Read the model definition and answer for the solid it produces. Units are mm, in the model's axes. Face numbers are marked on the shaded views. A direction names the side the tool comes from. Coordinates: 2 decimals unless noted, no trailing zeros. Loops run counter-clockwise (first coordinate to the right, second up) from the corner with the lowest first, then second, coordinate; pieces in that order, holes last.
Q1. Flat-ended cylindrical pins translate along their axes: P1, Ø1, axis at x = -11, y = -6, coming from the +Z side; P2, Ø5, axis at x = 12.5, y = -3, coming from the -Z side; P3, Ø0.9, axis at x = -21, y = 6.5, coming from the +Z side. Find the tip coordinate at first contact, or state that the pin passes through.
Q2. Section A-A (y = 0) is taken. Give the vertices of the cut face in (x, z) (3 decimals).
Q3. The mould has two halves that part along X. Classify the marked faces 1, 2 and 3: pulls with the +X half, pulls with the -X half, needs draft (parallel to the pull), parting line crosses it, or undercut.
Q4. Which of the six approach directions +Z, -Z, +X, -X, +Y, -Y give full straight-line access (tool end or side, diameter ignored) to the marked faces 4 and 5?
Q5. Section B-B (z = 0) is taken. Give the vertices of the cut face in (x, y) (3 decimals), then the cut area to 3 significant figures.
Q6. Section C-C (x = 24) is taken. Give the vertices of the cut face in (y, z).
Q7. Straight lines are drawn through the part: line 1 (X direction, y = 3.5, z = -4.25); line 2 (Z direction, x = 9, y = 0); line 3 (Z direction, x = 15.5, y = 0). For each, find the intervals that lie inside material, in ascending order.
Q8. Section D-D (z = 6) is taken. Give the vertices of the cut face in (x, y).
from build123d import *

# Parameters (mm, degrees)
F0_R      = 9
F1_DEPTH  = 14
F2_R      = 7.5
F3_DEPTH  = 15
F4_R      = 5
F5_DEPTH  = 10
F6_R      = 7.5
F7_DEPTH  = 11.5
F8_R      = 7.425
F9_DEPTH  = 1.5
F10_R     = 8
F11_DEPTH = 2
F13_DEPTH = 13.5


with BuildPart() as f1:
    # F0 (on Right) → F1 (new body, symmetric)
    with BuildSketch(Plane.YZ):
        Circle(F0_R)
    extrude(amount=F1_DEPTH, both=True)

    # F2 (on face) → F3 (join)
    with BuildSketch(Plane.YZ.offset(14)):
        Circle(F2_R)
    extrude(amount=F3_DEPTH)

    # F4 (on face) → F5 (join)
    with BuildSketch(Plane.YZ.offset(29)):
        Circle(F4_R)
    extrude(amount=F5_DEPTH)

    # F6 (on face) → F7 (join)
    with BuildSketch(Plane(origin=(-14, 0, 0), x_dir=(0, -1, 0), z_dir=(-1, 0, 0))):
        Circle(F6_R)
    extrude(amount=F7_DEPTH)

    # F8 (on face) → F9 (join)
    with BuildSketch(Plane(origin=(-25.5, 0, 0), x_dir=(0, -1, 0), z_dir=(-1, 0, 0))):
        Circle(F8_R)
    extrude(amount=F9_DEPTH)

    # F10 (on face) → F11 (join)
    with BuildSketch(Plane(origin=(-27, 0, 0), x_dir=(0, -1, 0), z_dir=(-1, 0, 0))):
        Circle(F10_R)
    extrude(amount=F11_DEPTH)

    # F12 (on face) → F13 (cut)
    with BuildSketch(Plane(origin=(-29, 0, 0), x_dir=(0, -1, 0), z_dir=(-1, 0, 0))):
        with BuildLine():
            Line((-7.8581168228, -1.5), (-4.8581168228, -1.5))
            Line((-4.8581168228, -1.5), (-4.8581168228, 1.5))
            Line((-4.8581168228, 1.5), (-7.8581168228, 1.5))
            add(Edge.make_bspline(
                [(-7.8581168228, 1.5), (-8.0546390686, 1), (-8.4476835604, 0), (-8.0546390686, -1), (-7.8581168228, -1.5)],
                knots=[0, 0, 0, 0, 0.5, 1, 1, 1, 1], degree=3))
        make_face()
    extrude(amount=-F13_DEPTH, mode=Mode.SUBTRACT)


solid = f1.part
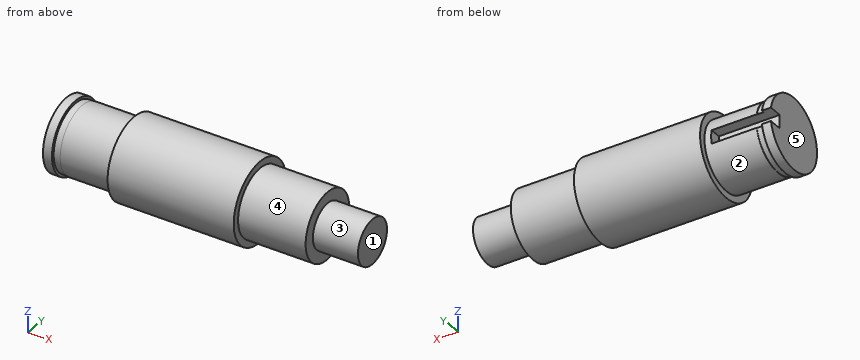
Numbers:
1. P1: stops at z = 7.12
1. P2: stops at z = -8.99
1. P3: stops at z = 4.43
2. outline: (-29, -8) - (-27, -8) - (-27, -7.425) - (-25.5, -7.425) - (-25.5, -7.5) - (-14, -7.5) - (-14, -9) - (14, -9) - (14, -7.5) - (29, -7.5) - (29, -5) - (39, -5) - (39, 5) - (29, 5) - (29, 7.5) - (14, 7.5) - (14, 9) - (-14, 9) - (-14, 7.5) - (-25.5, 7.5) - (-25.5, 7.425) - (-27, 7.425) - (-27, 8) - (-29, 8) - close
3. face 1: pulls with the +X half
3. face 2: undercut
3. face 3: needs draft
4. face 4: +X
4. face 5: +Z, -Z, -X, +Y, -Y
5. outline: (-29, -8) - (-27, -8) - (-27, -7.425) - (-25.5, -7.425) - (-25.5, -7.5) - (-14, -7.5) - (-14, -9) - (14, -9) - (14, -7.5) - (29, -7.5) - (29, -5) - (39, -5) - (39, 5) - (29, 5) - (29, 7.5) - (14, 7.5) - (14, 9) - (-14, 9) - (-14, 7.5) - (-15.5, 7.5) - (-15.5, 4.858) - (-29, 4.858) - close
5. area: 1,020 mm2
6. outline: circle Ø15 at (0, 0)
7. line 1: x = -29 to 29
7. line 2: z = -9 to 9
7. line 3: z = -7.5 to 7.5
8. outline: (-29, -5.29) - (-27, -5.29) - (-27, -4.37) - (-25.5, -4.37) - (-25.5, -4.5) - (-14, -4.5) - (-14, -6.71) - (14, -6.71) - (14, -4.5) - (29, -4.5) - (29, 4.5) - (14, 4.5) - (14, 6.71) - (-14, 6.71) - (-14, 4.5) - (-25.5, 4.5) - (-25.5, 4.37) - (-27, 4.37) - (-27, 5.29) - (-29, 5.29) - close
